Could you check a few things on this model? Use its own coordinates, in mm. A direction names the side the tool comes from. Coordinates: 2 decimals unless noted, no trailing zeros. Write each loop counter-clockwise with the first axis right and the second up, starting at its lowest first coordinate (ties: lowest second). Pieces come first, ordered by that corner, then holes.
```python
from build123d import *
from build123d.topology import SkipClean

# Parameters (mm, degrees)
SKETCH1_W           = 127
SKETCH1_H           = 76.2
BOSS_EXTRUDE1_DEPTH = 127
SHELL1_T            = -2.54
SKETCH2_W           = 132.08
SKETCH2_H           = 132.08
SKETCH2_W_2         = 127
SKETCH2_H_2         = 127
SKETCH2_W_3         = 121.92
SKETCH2_H_3         = 121.92
BOSS_EXTRUDE2_DEPTH = 25.4
SKETCH5_W           = 23.197534015
SKETCH5_H           = 57.422092124
CUT_EXTRUDE1_DEPTH  = 199.41286047
SKETCH6_W           = 45.064315034
SKETCH6_H           = 17.215386484
CUT_EXTRUDE2_DEPTH  = 199.41286047


with BuildPart() as part:
    # Sketch1 → Boss-Extrude1 (new body)
    with BuildSketch(Plane(origin=(0, 0, 0), x_dir=(1, 0, 0), z_dir=(0, 1, 0))):
        with Locations((-63.5, 38.1)):
            Rectangle(SKETCH1_W, SKETCH1_H)
    extrude(amount=BOSS_EXTRUDE1_DEPTH)

    # Shell1
    shell1_openings = [part.faces().sort_by_distance(p)[0] for p in [
        (-63.5, 63.5, 0),
    ]]
    offset(amount=SHELL1_T, openings=shell1_openings, kind=Kind.INTERSECTION)

    # Sketch2 → Boss-Extrude2 (add)
    # profile 1 of 2: a face of its own
    with BuildSketch(Plane.XY):
        with Locations((-63.5, 63.5)):
            Rectangle(SKETCH2_W, SKETCH2_H)
        with Locations((-63.5, 63.5)):
            Rectangle(SKETCH2_W_2, SKETCH2_H_2, mode=Mode.SUBTRACT)
    # profile 2 of 2: a face of its own
    with BuildSketch(Plane.XY):
        with Locations((-63.5, 63.5)):
            Rectangle(SKETCH2_W_2, SKETCH2_H_2)
        with Locations((-63.5, 63.5)):
            Rectangle(SKETCH2_W_3, SKETCH2_H_3, mode=Mode.SUBTRACT)
    extrude(amount=BOSS_EXTRUDE2_DEPTH)

    # Sketch3 → Cut-Revolve2 (revolve, cut)
    with SkipClean():  # the faces are left unmerged after this step: merging them gives an invalid solid
        with BuildSketch(Plane.ZY.offset(63.5)):
            with BuildLine():
                ThreePointArc((23.19621529, 63.5), (1013.79621529, -927.1), (2004.39621529, 63.5))
                Line((2004.39621529, 63.5), (23.19621529, 63.5))
            make_face()
            with BuildLine():
                Line((23.19621529, 63.5), (2004.39621529, 63.5))
                ThreePointArc((2004.39621529, 63.5), (1013.79621529, 1054.1), (23.19621529, 63.5))
            make_face()
        revolve(axis=Axis((-63.5, 63.5, 2004.39621529), (0, 0, -1)), mode=Mode.SUBTRACT)
    add(part.part.scale(1), mode=Mode.REPLACE)  # the faces are merged on a copy

    # Sketch5 → Cut-Extrude1 (cut, through all)
    with BuildSketch(Plane.ZY.offset(127)):
        with Locations((-52.940293684, 63.810930306)):
            Rectangle(SKETCH5_W, SKETCH5_H)
    extrude(amount=-CUT_EXTRUDE1_DEPTH, mode=Mode.SUBTRACT)

    # Sketch6 → Cut-Extrude2 (cut, through all)
    with BuildSketch(Plane.XZ):
        with Locations((-63.5, -55.050992996)):
            Rectangle(SKETCH6_W, SKETCH6_H)
    extrude(amount=-CUT_EXTRUDE2_DEPTH, mode=Mode.SUBTRACT)


solid = part.part
```
1. If we mould it in two halves opening along Y, with no side actions, what happens to faces 1 (the face through (-64, 127, -39)), 2 (the face through (-64, -2.54, 13)), 3 (the face through (-116, 1, 25.4)), 4 (the face through (-64, 124.46, -25))? For each: pulls with the +Y half, pulls with the -Y half, needs draft (parallel to the pull), parting line crosses it, or undercut.
Verdict:
face 1: pulls with the +Y half
face 2: pulls with the -Y half
face 3: needs draft
face 4: undercut
2. For pin 1 (12 mm diameter, centred on x = -100.5, z = -13, fed in from +Y); pin 2 (8 mm diameter, centred on y = 85, z = -32.5, fed in from -X); pin 3 (0.8 mm diameter, centred on x = -1.5, y = 71.5, fed in from +Z), each with a flat end and sliding along its axis, tell me the tip position at first contact or that it passes through.
Verdict:
pin 1: stops at y = 127
pin 2: stops at x = -127
pin 3: stops at z = 25.2
3. I want a section at C-C on x = -104.5. Please give me the cut outline in (y, z), plus the area to 3 significant figures.
Verdict:
outline: (-2.54, 0) - (0, 0) - (0, -76.2) - (127, -76.2) - (127, 0) - (129.54, 0) - (129.54, 25.4) - (124.46, 25.4) - (124.46, -73.66) - (2.54, -73.66) - (2.54, 25.4) - (-2.54, 25.4) - close
area: 955 mm2
4. Please list where these lines run through material, in increasing order: line 1 along X through (y, z) = (35, -39); line 2 along Y through (x, z) = (-121.5, -48); line 3 along Y through (x, z) = (-104.5, 11.5).
Verdict:
line 1: x = -127 to -124.46, -2.54 to 0
line 2: y = 0 to 2.54, 124.46 to 127
line 3: y = -2.54 to 2.54, 124.46 to 129.54
5. I want a section at A-A on z = -16. Please give me the cut outline in (x, y).
Verdict:
outline: (-127, 0) - (0, 0) - (0, 127) - (-127, 127) - close; hole (-124.46, 2.54) - (-2.54, 2.54) - (-2.54, 124.46) - (-124.46, 124.46) - close
6. On a 3-axis mill with a long thin cutter (end or side, diameter ignored), from which of +Z, -Z, +X, -X, +Y, -Y can I reach the whole of each face in a straight line? I mean faces 5 (the face through (0, 63, -38)), 6 (the face through (-64, 0, -39)), 7 (the face through (-64, 2.54, -25)). Say none if no direction works.
Verdict:
face 5: -Z, +X, +Y, -Y
face 6: -Z, +X, -X, -Y
face 7: +Z
7. I want a section at B-B on y = 69.5. Please give me the cut outline in (x, z).
Verdict:
outline: (-129.54, 0) - (-127, 0) - (-127, -41.34) - (-124.46, -41.34) - (-124.46, 25.09) arc R990.58 cw to (-129.27, 25.4) - (-129.54, 25.4) - close; (-127, -76.2) - (0, -76.2) - (0, -64.54) - (-2.54, -64.54) - (-2.54, -73.66) - (-124.46, -73.66) - (-124.46, -64.54) - (-127, -64.54) - close; (-2.54, -41.34) - (0, -41.34) - (0, 0) - (2.54, 0) - (2.54, 25.4) - (2.27, 25.4) arc R990.58 cw to (-2.54, 25.09) - close
8. I want a section at D-D on y = 96. Please give me the cut outline in (x, z), plus the area to 3 significant figures.
Verdict:
outline: (-129.54, 0) - (-127, 0) - (-127, -76.2) - (0, -76.2) - (0, 0) - (2.54, 0) - (2.54, 25.4) - (-2.54, 25.4) - (-2.54, -73.66) - (-124.46, -73.66) - (-124.46, 25.4) - (-129.54, 25.4) - close
area: 955 mm2
